from build123d import *

# Parameters (mm, degrees)
SKETCH2_W          = 6
SKETCH2_H          = 3
SKETCH3_W          = 20
SKETCH3_H          = 3
CUT_EXTRUDE1_DEPTH = 3


with BuildPart() as part:
    # Sketch1 → Revolve1 (revolve)
    with BuildSketch(Plane.XY, mode=Mode.PRIVATE) as revolve1_sk:
        Polygon((-110, 9.5), (-110, 12.5), (-100, 12.5), (-100, 9.5), (0, 9.5), (0, 0), (-130, 0), (-130, 9.5), align=None)
    revolve(revolve1_sk.sketch.rotate(Axis((0.866713413, 0, 0), (1, 0, 0)), 90), axis=Axis((0.866713413, 0, 0), (1, 0, 0)))

    # Sketch2 → Cut-Revolve1 (revolve, cut)
    with BuildSketch(Plane.XY, mode=Mode.PRIVATE) as cut_revolve1_sk:
        with Locations((-120, 8)):
            Rectangle(SKETCH2_W, SKETCH2_H)
    revolve(cut_revolve1_sk.sketch.rotate(Axis((-130, 0, 0), (1, 0, 0)), 90), axis=Axis((-130, 0, 0), (1, 0, 0)), mode=Mode.SUBTRACT)

    # Sketch3 → Cut-Extrude1 (cut, symmetric)
    with BuildSketch(Plane.XY):
        with Locations((-10, 8)):
            Rectangle(SKETCH3_W, SKETCH3_H)
    extrude(amount=CUT_EXTRUDE1_DEPTH, both=True, mode=Mode.SUBTRACT)


solid = part.part
Design review of the part built by this model. Coordinates are the model's own, in mm. A direction names the side the tool comes from. Round coordinates to 2 decimals unless told otherwise and drop trailing zeros. Loops run counter-clockwise (first coordinate to the right, second up) from the corner with the lowest first, then second, coordinate; pieces in that order, holes last. Notation, with made-up numbers: (61, 18) - (114, 18) arc R10 cw to (114, 36) - close; hole circle Ø3 at (-17.5, 73). An arc over 180 degrees is marked (long way). One line per item, written item: value. Start each with the question number.
1) Consider section B-B on y = 0. Give the boundary of the cut face in (x, z).
2) Insertion check: pin 1 Ø3 at (x, z) = (-89, 8) entering from -Y; pin 2 Ø10 at (x, y) = (-37, 0.5) entering from -Z; pin 3 Ø6 at (x, y) = (-69.5, 4.5) entering from +Z. Each pin has a flat end and moves straight along its axis. Give the tip position at first contact, or say it passes through.
3) For faces 4 (the cylindrical face through (-119.958, 3.955, -5.158)), 5 (the cylindrical face through (-49.3, -8.01, 5.11)), 6 (the cylindrical face through (-113.451, 9.274, -2.059)), 7 (the flat face through (-20, 8, 0)), list the 3-axis set-ups (+Z, -Z, +X, -X, +Y, -Y) from which the entire face can be reached by the end or side of a thin tool; tool diameter is ignored.
4) Consider section D-D on x = -41.5. Give the boundary of the cut face in (y, z), then the cut area to 3 significant figures.
5) To check wall thickness, follow L1, parallel to X at y = 0.75, z = 7.25; L2, parallel to X at y = -4.75, z = -10.75; L3, parallel to Y at x = -75.5, z = 0.5. State the ranges of each line that lie inside material, in increasing order. Write a range as from..to.
6) Consider section C-C on z = 0. Give the boundary of the cut face in (x, y), then the cut area to 3 significant figures.
7) Draft analysis for pull direction X (two halves, no side actions). For faces 1 (the flat face through (-10, 8, -3)), 2 (the flat face through (-117, 6, -4)), 3 (the flat face through (0, 0, 0)), state which applies: +X half, -X half, draft (parallel to the pull), parting line (faces both ways), or undercut.
8) Consider section A-A on z = 8. Give the boundary of the cut face in (x, y).
Reported:
1. outline: (-130, -9.5) - (-123, -9.5) - (-123, -6.5) - (-117, -6.5) - (-117, -9.5) - (-110, -9.5) - (-110, -12.5) - (-100, -12.5) - (-100, -9.5) - (0, -9.5) - (0, 9.5) - (-100, 9.5) - (-100, 12.5) - (-110, 12.5) - (-110, 9.5) - (-117, 9.5) - (-117, 6.5) - (-123, 6.5) - (-123, 9.5) - (-130, 9.5) - close
2. pin 1: stops at y = -6.93
2. pin 2: stops at z = -9.5
2. pin 3: stops at z = 9.38
3. face 4: none
3. face 5: +X
3. face 6: -X
3. face 7: +X, +Y
4. outline: circle Ø19 at (0, 0)
4. area: 284 mm^2
5. L1: x = -130..-123, -117..0
5. L2: x = -110..-100
5. L3: y = -9.49..9.49
6. outline: (-130, -9.5) - (-123, -9.5) - (-123, -6.5) - (-117, -6.5) - (-117, -9.5) - (-110, -9.5) - (-110, -12.5) - (-100, -12.5) - (-100, -9.5) - (0, -9.5) - (0, 6.5) - (-20, 6.5) - (-20, 9.5) - (-100, 9.5) - (-100, 12.5) - (-110, 12.5) - (-110, 9.5) - (-117, 9.5) - (-117, 6.5) - (-123, 6.5) - (-123, 9.5) - (-130, 9.5) - close
6. area: 2,430 mm^2
7. face 1: draft
7. face 2: undercut
7. face 3: +X half
8. outline: (-130, -5.12) - (-123, -5.12) - (-123, 5.12) - (-130, 5.12) - close; (-117, -5.12) - (-110, -5.12) - (-110, -9.6) - (-100, -9.6) - (-100, -5.12) - (0, -5.12) - (0, 5.12) - (-100, 5.12) - (-100, 9.6) - (-110, 9.6) - (-110, 5.12) - (-117, 5.12) - close
